from build123d import *

# Parameters (mm, degrees)
F1_DEPTH = 75
F4_DEPTH = 75.001
F7_DEPTH = 75
F9_D     = 15


with BuildPart() as f1:
    # F0 (on Front) → F1 (new body)
    with BuildSketch(Plane.XZ):
        Polygon((-50, 0), (0, 0), (50, 0), (50, 10.31), (-50, 10.31), align=None)
    extrude(amount=-F1_DEPTH)

    # F3 (on offset) → F4 (cut, through all)
    with BuildSketch(Plane.XZ):
        Polygon((-15, 0), (0, 0), (15, 0), (15, 3), (-15, 3), align=None)
    extrude(amount=-F4_DEPTH, mode=Mode.SUBTRACT)

    # F6 (on offset) → F7 (join)
    with BuildSketch(Plane.XZ):
        Polygon((-15, 10.31), (0, 10.31), (15, 10.31), (15, 13.31), (-15, 13.31), align=None)
    extrude(amount=-F7_DEPTH)

    # F9 (through all)
    with Locations(Plane(origin=(0, 0, 0), x_dir=(1, 0, 0), z_dir=(0, 0, -1))):
        with Locations((-34, -61), (-34, -16), (36, -61), (36, -16)):
            Hole(F9_D / 2)


solid = f1.part
For this review, take the finished solid that the model builds, in its own axes (mm). A direction names the side the tool comes from. Round coordinates to 2 decimals unless told otherwise and drop trailing zeros. Loops run counter-clockwise (first coordinate to the right, second up) from the corner with the lowest first, then second, coordinate; pieces in that order, holes last. Notation, with made-up numbers: (88, -15) - (125, -15) arc R12 cw to (125, 0) - close; hole circle Ø6 at (-33.75, 46). An arc over 180 degrees is marked (long way). Use one line per item in the form item = value.
Item 1: Clearance check with flat-ended pins moving along their axes: P1, Ø1.5, axis at y = 51, z = 12.5, coming from the +X side; P2, Ø17.5, axis at x = -35.5, y = 38.5, coming from the +Z side; P3, Ø3.5, axis at y = 19.5, z = 12.5, coming from the -X side. State where each tip first meets the part, or that it passes through.
Answers:
P1 = 15
P2 = 10.31
P3 = -15
Item 2: Tool access review of faces 1 (the flat face through (-15, 37, 2)), 2 (the flat face through (-32, 37, 10.31)), 3 (the flat face through (15, 37, 12)), 4 (the flat face through (50, 37, 5)): name each direction out of +Z, -Z, +X, -X, +Y, -Y from which nothing blocks a thin tool from reaching the whole face with its end or side.
Answers:
face_1 = -Z, +Y, -Y
face_2 = +Z, -X, +Y, -Y
face_3 = +Z, +X, +Y, -Y
face_4 = +Z, -Z, +X, +Y, -Y
Item 3: Consider section C-C on y = 44. Write out the cut boundary in (x, z), then the cut area to 3 significant figures.
Answers:
outline = (-50, 0) - (-15, 0) - (-15, 3) - (15, 3) - (15, 0) - (50, 0) - (50, 10.31) - (15, 10.31) - (15, 13.31) - (-15, 13.31) - (-15, 10.31) - (-50, 10.31) - close
area = 1,030 mm^2
Item 4: Consider section A-A on y = 16. Write out the cut boundary in (x, z), then the cut area to 3 significant figures.
Answers:
outline = (-50, 0) - (-41.5, 0) - (-41.5, 10.31) - (-50, 10.31) - close; (-26.5, 0) - (-15, 0) - (-15, 3) - (15, 3) - (15, 0) - (28.5, 0) - (28.5, 10.31) - (15, 10.31) - (15, 13.31) - (-15, 13.31) - (-15, 10.31) - (-26.5, 10.31) - close; (43.5, 0) - (50, 0) - (50, 10.31) - (43.5, 10.31) - close
area = 722 mm^2
Item 5: Mouldability with a two-part tool opening along X and no side actions: class faces 5 (the flat face through (-1, 0, 7)), 6 (the cylindrical face through (-28.5, 55.9, 5.2)), 7 (the flat face through (-50, 37, 5)) as +X half, -X half, draft (parallel to the pull), parting line (faces both ways), or undercut.
Answers:
face_5 = draft
face_6 = undercut
face_7 = -X half
Item 6: For line 1 (Y direction, x = -34, z = 5.75); line 2 (X direction, y = 61, z = 3.5); line 3 (X direction, y = 60, z = 5.5), list the stretches that pass through material, from the lowest coordinate up.
Answers:
line_1 = 0 to 8.5, 23.5 to 53.5, 68.5 to 75
line_2 = -50 to -41.5, -26.5 to 28.5, 43.5 to 50
line_3 = -50 to -41.43, -26.57 to 28.57, 43.43 to 50
Item 7: Consider section D-D on x = 36. Write out the cut boundary in (y, z), then the cut area to 3 significant figures.
Answers:
outline = (0, 0) - (8.5, 0) - (8.5, 10.31) - (0, 10.31) - close; (23.5, 0) - (53.5, 0) - (53.5, 10.31) - (23.5, 10.31) - close; (68.5, 0) - (75, 0) - (75, 10.31) - (68.5, 10.31) - close
area = 464 mm^2
Item 8: Consider section B-B on x = -37. Write out the cut boundary in (y, z), then the cut area to 3 significant figures.
Answers:
outline = (0, 0) - (9.13, 0) - (9.13, 10.31) - (0, 10.31) - close; (22.87, 0) - (54.13, 0) - (54.13, 10.31) - (22.87, 10.31) - close; (67.87, 0) - (75, 0) - (75, 10.31) - (67.87, 10.31) - close
area = 490 mm^2
